from build123d import *

# Parameters (mm, degrees)
SKETCH5_W           = 59.5
SKETCH5_H           = 59.5
SKETCH5_W_2         = 52.5
SKETCH5_H_2         = 52.5
BOSS_EXTRUDE5_DEPTH = 50
SKETCH7_R           = 1.75
BOSS_EXTRUDE7_DEPTH = 4


with BuildPart() as part:
    # Sketch5 → Boss-Extrude5 (new body)
    with BuildSketch(Plane.XY):
        with Locations((26.25, 26.25)):
            Rectangle(SKETCH5_W, SKETCH5_H)
        with Locations((26.25, 26.25)):
            Rectangle(SKETCH5_W_2, SKETCH5_H_2, mode=Mode.SUBTRACT)
    extrude(amount=BOSS_EXTRUDE5_DEPTH)

    # Sketch7 → Boss-Extrude7 (add)
    with BuildSketch(Plane.XZ.offset(3.5)):
        Polygon((-3.5, 50), (-18.5, 50), (-18.5, 0), (71, 0), (71, 50), (56, 50), align=None)
        with Locations(Location((-11, 42.5, 0), (0, 0, 270))):
            Circle(SKETCH7_R, mode=Mode.SUBTRACT)
        with Locations(Location((-11, 7.5, 0), (0, 0, 270))):
            Circle(SKETCH7_R, mode=Mode.SUBTRACT)
        with Locations(Location((63.5, 7.5, 0), (0, 0, 90))):
            Circle(SKETCH7_R, mode=Mode.SUBTRACT)
        with Locations(Location((63.5, 42.5, 0), (0, 0, 90))):
            Circle(SKETCH7_R, mode=Mode.SUBTRACT)
    extrude(amount=-BOSS_EXTRUDE7_DEPTH)


solid = part.part
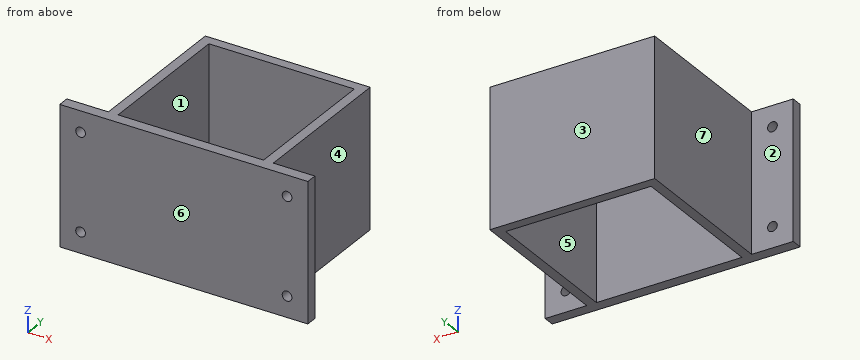
Design review of the part built by this model. Coordinates are the model's own, in mm. Face numbers are marked on the shaded views. A direction names the side the tool comes from. Round coordinates to 2 decimals unless told otherwise and drop trailing zeros. Order: outer loops, then holes, each group sorted by start corner. A loop starts at its lowest first (then second) coordinate and runs counter-clockwise, first axis right, second up. Notation, with made-up numbers: M 17,15.25 L 48,15.25 A28 ccw 48,54.25 Z; hole C 56.5,-32.75 d6. An arc over 180 degrees is marked long. Answer as CSV lines item,"result". Start each with the question number.
1) The part is to be moulded in two halves that separate along Y. For the marked faces 5, 6 and 7, say which applies: +Y half, -Y half, draft (parallel to the pull), parting line (faces both ways), or undercut.
2) Add section C-C (z = 23.5). Give the boundary of the cut face in (x, y), then the cut area to 3 significant figures.
3) Tool access review of the marked faces 1, 2, 3 and 4: name each direction out of +Z, -Z, +X, -X, +Y, -Y from which nothing blocks a thin tool from reaching the whole face with its end or side.
4) Add section B-B (x = -11). Give the boundary of the cut face in (y, z).
5) Wall thickness on line 1 along Z through (x, y) = (63.5, -1.75); line 2 along X through (y, z) = (-0.5, 42.5); line 3 along X through (y, z) = (29.5, 35.5): over which ranges is each line inside the solid? List them lowest first. Write a range as [from, to].
6) Add section A-A (z = 42.5). Give the boundary of the cut face in (x, y).
7) Add section D-D (y = 44.5). Give the boundary of the cut face in (x, z).
8) For pin 1 Ø7.5 at (x, z) = (67, 31) entering from +Y; pin 2 Ø2 at (y, z) = (38, 11.5) entering from +X; pin 3 Ø8 at (y, z) = (21.5, 7.5) entering from -X, all flat-tipped, find the tip position at first contact; note any pin that passes through.
Resolved:
1,face 5,"undercut"
1,face 6,"-Y half"
1,face 7,"draft"
2,outline,"M -18.5,-3.5 L 71,-3.5 L 71,0.5 L 56,0.5 L 56,56 L -3.5,56 L -3.5,0.5 L -18.5,0.5 Z; hole M 0,0.5 L 52.5,0.5 L 52.5,52.5 L 0,52.5 Z"
2,area,"930 mm^2"
3,face 1,"+Z, -Z"
3,face 2,"+Z, -Z, -X, +Y"
3,face 3,"+Z, -Z, +X, -X, +Y"
3,face 4,"+Z, -Z, +X, +Y"
4,outline,"M -3.5,0 L 0.5,0 L 0.5,5.75 L -3.5,5.75 Z; M -3.5,9.25 L 0.5,9.25 L 0.5,40.75 L -3.5,40.75 Z; M -3.5,44.25 L 0.5,44.25 L 0.5,50 L -3.5,50 Z"
5,line 1,"[0, 5.75], [9.25, 40.75], [44.25, 50]"
5,line 2,"[-18.5, -12.75], [-9.25, 61.75], [65.25, 71]"
5,line 3,"[-3.5, 0], [52.5, 56]"
6,outline,"M -18.5,-3.5 L -12.75,-3.5 L -12.75,0.5 L -18.5,0.5 Z; M -9.25,-3.5 L 61.75,-3.5 L 61.75,0.5 L 56,0.5 L 56,56 L -3.5,56 L -3.5,0.5 L -9.25,0.5 Z; M 65.25,-3.5 L 71,-3.5 L 71,0.5 L 65.25,0.5 Z; hole M 0,0.5 L 52.5,0.5 L 52.5,52.5 L 0,52.5 Z"
7,outline,"M -3.5,0 L 0,0 L 0,50 L -3.5,50 Z; M 52.5,0 L 56,0 L 56,50 L 52.5,50 Z"
8,pin 1,"y = 0.5"
8,pin 2,"x = 56"
8,pin 3,"x = -3.5"
